Work out the finished part from the listing and answer in its coordinate system (mm). A direction names the side the tool comes from. Give positions to 0.01 mm unless a question says otherwise; leave off trailing zeros. Write each loop counter-clockwise with the first axis right and the second up, starting at its lowest first coordinate (ties: lowest second). Pieces come first, ordered by that corner, then holes. Notation, with made-up numbers: (-13.75, 2.5) -> (36.25, 2.5) arc R21 ccw to (36.25, 8.5) -> close; hole circle Ø1 at (47.5, -34.75). An arc over 180 degrees is marked (long way). Use a Markdown table: item, result. Add a question column.
Q1. Section A-A, the plane x = -107.5 is taken. Give the vertices of the cut face in (y, z).
Q2. Section B-B, the plane z = -30.5 is taken. Give the vertices of the cut face in (x, y).
Q3. Consider line 1 (X direction, y = 1.75, z = -7.5); line 2 (Y direction, x = -68, z = -62); line 3 (X direction, y = 4.5, z = -28). Determine where each line is inside the solid, lowest interval first.
Q4. Each of these flat-tipped pins is pushed along its axis until it touches: pin 1 Ø5 at (y, z) = (11, -71.5) entering from -X; pin 2 Ø10 at (x, z) = (-86.5, -37) entering from -Y; pin 3 Ø4 at (x, y) = (-66, 9.5) entering from +Z; pin 4 Ø3 at (x, z) = (-37, -27) entering from -Y. Where does it stop, or does it pass through?
Q5. For faces 4 (the face through (-60.714, 2.004, -47.454)), 5 (the face through (-176.797, 6.605, -11.434)), 6 (the face through (-43.18, 7, -15)), 7 (the face through (-103, 2, -14.732)), determine the directions among +Z, -Z, +X, -X, +Y, -Y from which every point of the face is accessible in a straight line to the end or side of a thin tool.
Q6. Section D-D, the plane z = -59 is taken. Give the vertices of the cut face in (x, y).
Q7. Section C-C, the plane y = 17.75 is taken. Give the vertices of the cut face in (x, z), plus the area to 3 significant figures.
Q8. For a pull along Z with two mould halves and no side action, classify faces 1 (the face through (-111.87, 10.5, -50.09)), 2 (the face through (-112, 0, -73)), 3 (the face through (-145.452, 2.004, -9.95)) as pulls with the +Z half, pulls with the -Z half, needs draft (parallel to the pull), parting line crosses it, or undercut.
from build123d import *

# Parameters (mm, degrees)
BOSS_EXTRUDE1_DEPTH = 195.58
SKETCH2_R           = 3.3147
CUT_EXTRUDE1_DEPTH  = 38.1
SKETCH3_W           = 27.94
SKETCH3_H           = 4.064
CUT_EXTRUDE2_DEPTH  = 405.649982083
CUT_EXTRUDE3_DEPTH  = 4.064
SKETCH7_W           = 101.6
SKETCH7_H           = 20.540040578
CUT_EXTRUDE5_DEPTH  = 226.06
CUT_EXTRUDE6_DEPTH  = 4.064
SKETCH10_R          = 1.905
SKETCH10_R_2        = 1.949893387
CUT_EXTRUDE7_DEPTH  = 12.7


with BuildPart() as part:
    # Sketch1 → Boss-Extrude1 (new, symmetric)
    with BuildSketch(Plane(origin=(0, 0, 0), x_dir=(0, 0, -1), z_dir=(1, 0, 0))):
        Polygon((0, 0), (0, 20.32), (101.6, 0.4), (101.6, 0), align=None)
    extrude(amount=BOSS_EXTRUDE1_DEPTH, both=True)

    # Sketch2 → Cut-Extrude1 (cut)
    with BuildSketch(Plane(origin=(195.58, 0, 0), x_dir=(0, 0, -1), z_dir=(1, 0, 0))):
        with Locations((9.652, 3.81)):
            Circle(SKETCH2_R)
        with Locations((47.752, 3.81)):
            Circle(SKETCH2_R)
    cut_extrude1 = extrude(amount=-CUT_EXTRUDE1_DEPTH, mode=Mode.SUBTRACT)

    # Mirror3: Cut-Extrude1 across plane
    add(cut_extrude1.mirror(Plane(origin=(0, 0, 0), x_dir=(0, 0, 1), z_dir=(1, 0, 0))), mode=Mode.SUBTRACT)

    # Sketch3 → Cut-Extrude2 (cut, through all)
    with BuildSketch(Plane.ZY.offset(195.58)):
        with Locations((-28.702, 2.032)):
            Rectangle(SKETCH3_W, SKETCH3_H)
    extrude(amount=-CUT_EXTRUDE2_DEPTH, mode=Mode.SUBTRACT)

    # Sketch4 → Cut-Extrude3 (cut)
    with BuildSketch(Plane.XZ):
        Polygon((-144.78, -42.672), (-146.105623787, -52.104303355), (-144.78, -52.104303355), (-128.584447573, -52.104303355), (-127.258823787, -52.104303355), (-128.584447573, -42.672), align=None)
        Polygon((-77.581247573, -42.672), (-78.90687136, -52.104303355), (-77.581247573, -52.104303355), (-61.385695147, -52.104303355), (-60.06007136, -52.104303355), (-61.385695147, -42.672), align=None)
        Polygon((-10.382495147, -42.672), (-11.708118933, -52.104303355), (-10.382495147, -52.104303355), (5.81305728, -52.104303355), (7.138681067, -52.104303355), (5.81305728, -42.672), align=None)
        Polygon((56.81625728, -42.672), (55.490633493, -52.104303355), (56.81625728, -52.104303355), (73.011809707, -52.104303355), (74.337433493, -52.104303355), (73.011809707, -42.672), align=None)
        Polygon((124.015009707, -42.672), (122.68938592, -52.104303355), (124.015009707, -52.104303355), (140.210562134, -52.104303355), (141.53618592, -52.104303355), (140.210562134, -42.672), align=None)
        Polygon((124.015009707, -14.732), (140.210562134, -14.732), (141.53618592, -5.299696645), (140.210562134, -5.299696645), (124.015009707, -5.299696645), (122.68938592, -5.299696645), align=None)
        Polygon((56.81625728, -14.732), (73.011809707, -14.732), (74.337433493, -5.299696645), (73.011809707, -5.299696645), (56.81625728, -5.299696645), (55.490633493, -5.299696645), align=None)
        Polygon((-10.382495147, -14.732), (5.81305728, -14.732), (7.138681067, -5.299696645), (5.81305728, -5.299696645), (-10.382495147, -5.299696645), (-11.708118933, -5.299696645), align=None)
        Polygon((-77.581247573, -14.732), (-61.385695147, -14.732), (-60.06007136, -5.299696645), (-61.385695147, -5.299696645), (-77.581247573, -5.299696645), (-78.90687136, -5.299696645), align=None)
        Polygon((-144.78, -14.732), (-128.584447573, -14.732), (-127.258823787, -5.299696645), (-128.584447573, -5.299696645), (-144.78, -5.299696645), (-146.105623787, -5.299696645), align=None)
    extrude(amount=-CUT_EXTRUDE3_DEPTH, mode=Mode.SUBTRACT)

    # Sketch7 → Cut-Extrude5 (cut)
    with BuildSketch(Plane(origin=(195.58, 0, 0), x_dir=(0, 0, -1), z_dir=(1, 0, 0))):
        with Locations((50.8, 10.270020289)):
            Rectangle(SKETCH7_W, SKETCH7_H)
    extrude(amount=-CUT_EXTRUDE5_DEPTH, mode=Mode.SUBTRACT)

    # Sketch9 → Cut-Extrude6 (cut)
    with BuildSketch(Plane.XZ.offset(-4.064)):
        Polygon((-30.48, -20.447), (-39.912303355, -19.121376213), (-39.912303355, -38.171376213), (-30.48, -36.845752427), align=None)
    extrude(amount=-CUT_EXTRUDE6_DEPTH, mode=Mode.SUBTRACT)

    # Sketch10 → Cut-Extrude7 (cut)
    with BuildSketch(Plane(origin=(-30.48, 0, 0), x_dir=(0, 0, -1), z_dir=(1, 0, 0))):
        with Locations((15.24, 6.604)):
            Circle(SKETCH10_R)
        with Locations((45.72, 6.604)):
            Circle(SKETCH10_R_2)
    extrude(amount=-CUT_EXTRUDE7_DEPTH, mode=Mode.SUBTRACT)


solid = part.part
Result set:
| question | item | result |
|---|---|---|
| 1 | outline | (0, -101.6) -> (0.4, -101.6) -> (20.32, 0) -> (0, 0) -> (0, -14.73) -> (4.06, -14.73) -> (4.06, -42.67) -> (0, -42.67) -> close |
| 2 | outline | (-195.58, 4.06) -> (-39.91, 4.06) -> (-39.91, 8.13) -> (-30.48, 8.13) -> (-30.48, 14.34) -> (-195.58, 14.34) -> close |
| 3 | line 1 | x = -157.48 to -145.8, -127.57 to -78.6, -60.37 to -30.48 |
| 3 | line 2 | y = 0 to 8.16 |
| 3 | line 3 | x = -195.58 to -39.91 |
| 4 | pin 1 | passes through |
| 4 | pin 2 | stops at y = 4.06 |
| 4 | pin 3 | stops at z = 0 |
| 4 | pin 4 | stops at y = 8.13 |
| 5 | face 4 | -Y |
| 5 | face 5 | -X |
| 5 | face 6 | +X |
| 5 | face 7 | +X, -X, -Y |
| 6 | outline | (-195.58, 0) -> (-30.48, 0) -> (-30.48, 8.75) -> (-195.58, 8.75) -> close |
| 7 | outline | (-195.58, -13.11) -> (-30.48, -13.11) -> (-30.48, 0) -> (-195.58, 0) -> close |
| 7 | area | 2,160 mm2 |
| 8 | face 1 | pulls with the -Z half |
| 8 | face 2 | needs draft |
| 8 | face 3 | undercut |
